Can you work these out from the model? Positions are in its coordinate system, mm. Face numbers are marked on the shaded views. Give positions to 0.01 mm unless a question says otherwise; leave off trailing zeros. Order: outer loops, then holes, each group sorted by start corner. A loop starts at its lowest first (then second) coordinate and runs counter-clockwise, first axis right, second up. Notation, with made-up numbers: (83.5, 21) - (88.5, 21) arc R22 cw to (88.5, 50) - close; hole circle Ø7 at (31.5, 39.25). An arc over 180 degrees is marked (long way). Answer as CSV lines item,"result".
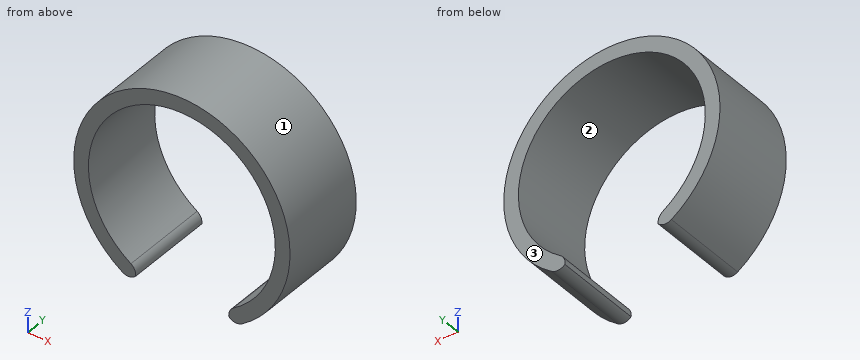
```python
from build123d import *

# Parameters (mm, degrees)
F1_DEPTH    = 8.5
F2_T1_DEPTH = 13.246827309
F2_T3_DEPTH = 14.0456784574


# Not quite as in the source:
# - a fillet or chamfer that OpenCascade refuses, or shapes differently, is made with other operations: its cross-section is extruded or revolved along the edge and cut away or added


with BuildPart() as f1:
    # F0 (on Front) → F1 (new body)
    with BuildSketch(Plane.XZ):
        with BuildLine():
            ThreePointArc((-4.0781486701, -7.910670226), (-0.0323602773, 8.899941169), (4.1355666361, -7.880805073))
            Line((4.1355666361, -7.880805073), (4.7861052081, -9.1204822755))
            ThreePointArc((4.7861052081, -9.1204822755), (-0.037450658, 10.2999319147), (-4.7196552025, -9.1550453177))
            Line((-4.7196552025, -9.1550453177), (-4.0781486701, -7.910670226))
        make_face()
    extrude(amount=F1_DEPTH)

    # F2: fillet of radius 1 on 4 edges, made by hand

    # F2_s2 → F2_t1 (cut)
    with BuildSketch(Plane.XZ.offset(-2.3734136545)):
        with BuildLine():
            ThreePointArc((-4.8563481702, -7.4582761044), (-4.4353117021, -8.0403480428), (-4.5131659168, -8.7545036072))
            Line((-4.5131659168, -8.7545036072), (-4.0781486701, -7.910670226))
            ThreePointArc((-4.0781486701, -7.910670226), (-4.4729714461, -7.6943178023), (-4.8563481702, -7.4582761044))
        make_face()
        with BuildLine():
            ThreePointArc((4.9104557842, -7.4227639051), (4.4936632318, -8.0078821984), (4.5767086731, -8.72145273))
            Line((4.5767086731, -8.72145273), (4.1355666361, -7.880805073))
            ThreePointArc((4.1355666361, -7.880805073), (4.5288056742, -7.6615872484), (4.9104557842, -7.4227639051))
        make_face()
    extrude(amount=F2_T1_DEPTH, mode=Mode.SUBTRACT)

    # F2_s4 → F2_t3 (cut)
    with BuildSketch(Plane.XZ.offset(-2.7728392287)):
        with BuildLine():
            ThreePointArc((4.2963798875, -8.1872534993), (4.9361379588, -8.6919225089), (5.7390532384, -8.5529683693))
            ThreePointArc((5.7390532384, -8.5529683693), (5.2702237229, -8.849561679), (4.7861052081, -9.1204822755))
            Line((4.7861052081, -9.1204822755), (4.2963798875, -8.1872534993))
        make_face()
        with BuildLine():
            ThreePointArc((-5.6767049543, -8.5944761831), (-4.8728004404, -8.7275879094), (-4.2367291997, -8.2182799714))
            Line((-4.2367291997, -8.2182799714), (-4.7196552025, -9.1550453177))
            ThreePointArc((-4.7196552025, -9.1550453177), (-5.2057310309, -8.8876523579), (-5.6767049543, -8.5944761831))
        make_face()
    extrude(amount=F2_T3_DEPTH, mode=Mode.SUBTRACT)


solid = f1.part
```
1) I want a section at B-B on x = -7.5. Write out the boundary of the cut face in (y, z).
Answer block:
outline,"(-8.5, -7.06) - (0, -7.06) - (0, -4.79) - (-8.5, -4.79) - close; (-8.5, 4.79) - (0, 4.79) - (0, 7.06) - (-8.5, 7.06) - close"
2) If we mould it in two halves opening along X, with no side actions, what happens to the marked faces 1, 2 and 3? For each: +X half, -X half, draft (parallel to the pull), parting line (faces both ways), or undercut.
Answer block:
face 1,"parting line"
face 2,"undercut"
face 3,"draft"
3) I want a section at D-D on y = -4.5. Write out the boundary of the cut face in (x, z).
Answer block:
outline,"(-5.68, -8.59) arc R1 ccw to (-4.42, -8.47) arc R1 ccw to (-4.86, -7.46) arc R8.9 cw (long way) to (4.91, -7.42) arc R1 ccw to (4.48, -8.43) arc R1 ccw to (5.74, -8.55) arc R10.3 ccw (long way) to start"
4) I want a section at A-A on z = 0. Write out the boundary of the cut face in (x, y), plus the area to 3 significant figures.
Answer block:
outline,"(-10.3, -8.5) - (-8.9, -8.5) - (-8.9, 0) - (-10.3, 0) - close; (8.9, -8.5) - (10.3, -8.5) - (10.3, 0) - (8.9, 0) - close"
area,"23.8 mm2"
5) I want a section at C-C on x = 0. Write out the boundary of the cut face in (y, z).
Answer block:
outline,"(-8.5, 8.9) - (0, 8.9) - (0, 10.3) - (-8.5, 10.3) - close"
6) I'm going to push flat-ended pins straight in: P1, Ø1.5, axis at y = -7, z = -7, coming from the -X side; P2, Ø1, axis at y = -2.5, z = -5, coming from the +X side (3 decimals). Where does each tip first touch, or does it pass through?
Answer block:
P1,"x = -8.19"
P2,"x = 9.265"
7) I need wall thicknesses on line 1 along X through (y, z) = (-4, 0); line 2 along X through (y, z) = (-4.25, 4.25); line 3 along Z through (x, y) = (0, -6). Which ranges of each line are inside material? Lowest first, please. Write a range as [from, to].
Answer block:
line 1,"[-10.3, -8.9], [8.9, 10.3]"
line 2,"[-9.38, -7.82], [7.82, 9.38]"
line 3,"[8.9, 10.3]"
